Here's how the part is built. I have some questions about the finished solid (model axes, mm). A direction names the side the tool comes from. Give positions to 0.01 mm unless a question says otherwise; leave off trailing zeros. Write each loop counter-clockwise with the first axis right and the second up, starting at its lowest first coordinate (ties: lowest second). Pieces come first, ordered by that corner, then holes. Notation, with made-up numbers: (17, 47) -> (39, 47) arc R24 cw to (39, 59) -> close; hole circle Ø1 at (48.25, 82). An arc over 180 degrees is marked (long way). Use CSV: the item, a comma, the result in double quotes. Start each with the question number.
(1) Suppose I cut it at C-C on z = 0.6. List the corners of the cut face in (x, y) for me, plus the area to 3 significant figures.
(2) Which directions (+Z, -Z, +X, -X, +Y, -Y) give clear straight access to the entire face, cutting with the end or side of a thin tool? Please do faces 4 (the flat face through (7, 127.05, 1)), 5 (the flat face through (14.9, 63, 1)).
(3) Suppose I cut it at A-A on y = 39.2. List the corners of the cut face in (x, z) for me.
(4) If we mould it in two halves opening along X, with no side actions, what happens to faces 1 (the flat face through (7, 0, 1)), 2 (the flat face through (7, 123.75, 1)), 3 (the flat face through (0, 63, 1))? For each: pulls with the +X half, pulls with the -X half, needs draft (parallel to the pull), parting line crosses it, or undercut.
(5) Suppose I cut it at B-B on x = 7.45. List the corners of the cut face in (y, z) for me, plus the area to 4 significant figures.
(6) I need wall thicknesses on L1, parallel to Y at x = 9.75, z = 2.15; L2, parallel to X at y = 40, z = 1.25. Which ranges of each line are inside material? Lowest first, please. Write a range as [from, to].
from build123d import *

# Parameters (mm, degrees)
MODEL_W                 = 14.9
MODEL_H                 = 128.4
BOSS_EXTRU_1_DEPTH      = 2.5
ESQUISSE1_R             = 1.4
ESQUISSE1_R_2           = 2
ENL_V_MAT_EXTRU_1_DEPTH = 130.285807419


with BuildPart() as part:
    # Model → Boss.-Extru.1 (new body)
    with BuildSketch(Plane.XY):
        with Locations((7.45, 64.2)):
            Rectangle(MODEL_W, MODEL_H)
        with BuildLine():
            Line((9.895403852, 123.75), (5.004596148, 123.75))
            ThreePointArc((5.004596148, 123.75), (4.5, 125.4), (5.004596148, 127.05))
            Line((5.004596148, 127.05), (9.895403852, 127.05))
            ThreePointArc((9.895403852, 127.05), (10.4, 125.4), (9.895403852, 123.75))
        make_face(mode=Mode.SUBTRACT)
        with BuildLine():
            Line((9.895403852, 1.35), (5.004596148, 1.35))
            ThreePointArc((5.004596148, 1.35), (4.5, 3), (5.004596148, 4.65))
            Line((5.004596148, 4.65), (9.895403852, 4.65))
            ThreePointArc((9.895403852, 4.65), (10.4, 3), (9.895403852, 1.35))
        make_face(mode=Mode.SUBTRACT)
    extrude(amount=BOSS_EXTRU_1_DEPTH)

    # Esquisse1 → Enlèv. mat.-Extru.1 (cut, through all)
    with BuildSketch(Plane.XY.offset(2.5)):
        with Locations((7.45, 63.2)):
            Circle(ESQUISSE1_R)
        with Locations((7.45, 51.2)):
            Circle(ESQUISSE1_R)
        with Locations((7.45, 39.2)):
            Circle(ESQUISSE1_R)
        with Locations((7.45, 27.2)):
            Circle(ESQUISSE1_R_2)
    extrude(amount=-ENL_V_MAT_EXTRU_1_DEPTH, mode=Mode.SUBTRACT)


solid = part.part
Geometry says:
1,outline,"(0, 0) -> (14.9, 0) -> (14.9, 128.4) -> (0, 128.4) -> close; hole (5, 1.35) -> (9.9, 1.35) arc R2.95 ccw to (9.9, 4.65) -> (5, 4.65) arc R2.95 ccw to start; hole (5, 123.75) -> (9.9, 123.75) arc R2.95 ccw to (9.9, 127.05) -> (5, 127.05) arc R2.95 ccw to start; hole circle Ø4 at (7.45, 27.2); hole circle Ø2.8 at (7.45, 39.2); hole circle Ø2.8 at (7.45, 51.2); hole circle Ø2.8 at (7.45, 63.2)"
1,area,"1,850 mm²"
2,face 4,"+Z, -Z"
2,face 5,"+Z, -Z, +X, +Y, -Y"
3,outline,"(0, 0) -> (6.05, 0) -> (6.05, 2.5) -> (0, 2.5) -> close; (8.85, 0) -> (14.9, 0) -> (14.9, 2.5) -> (8.85, 2.5) -> close"
4,face 1,"needs draft"
4,face 2,"undercut"
4,face 3,"pulls with the -X half"
5,outline,"(0, 0) -> (1.35, 0) -> (1.35, 2.5) -> (0, 2.5) -> close; (4.65, 0) -> (25.2, 0) -> (25.2, 2.5) -> (4.65, 2.5) -> close; (29.2, 0) -> (37.8, 0) -> (37.8, 2.5) -> (29.2, 2.5) -> close; (40.6, 0) -> (49.8, 0) -> (49.8, 2.5) -> (40.6, 2.5) -> close; (52.6, 0) -> (61.8, 0) -> (61.8, 2.5) -> (52.6, 2.5) -> close; (64.6, 0) -> (123.75, 0) -> (123.75, 2.5) -> (64.6, 2.5) -> close; (127.05, 0) -> (128.4, 0) -> (128.4, 2.5) -> (127.05, 2.5) -> close"
5,area,"273.5 mm²"
6,L1,"[0, 1.35], [4.65, 123.75], [127.05, 128.4]"
6,L2,"[0, 6.3], [8.6, 14.9]"
